```python
from build123d import *

# Parameters (mm, degrees)
F0_W     = 4.5
F0_H     = 30
F0_W_2   = 4
F1_DEPTH = 5
F2_DEPTH = 10
F3_R     = 3
F4_R     = 1
F6_DEPTH = 30


with BuildPart() as f1:
    # F0 (on Top) → F1 (new body)
    with BuildSketch(Plane.XY):
        with Locations((-4.7856509686, -8.5439818352)):
            Rectangle(F0_W, F0_H)
        with Locations((-9.0356509686, -8.5439818352)):
            Rectangle(F0_W_2, F0_H)
        with Locations((-0.5356509686, -8.5439818352)):
            Rectangle(F0_W_2, F0_H)
    extrude(amount=-F1_DEPTH)

    # F0 (on Top) → F2 (join)
    with BuildSketch(Plane.XY):
        with Locations((-9.0356509686, -8.5439818352)):
            Rectangle(F0_W_2, F0_H)
        with Locations((-0.5356509686, -8.5439818352)):
            Rectangle(F0_W_2, F0_H)
    extrude(amount=F2_DEPTH)

    # F3
    f3_edges = [f1.edges().sort_by_distance(p)[0] for p in [
        (1.464349, -8.543982, -5),
        (-11.035651, -8.543982, -5),
    ]]
    fillet(f3_edges, radius=F3_R)

    # F4
    f4_edges = [f1.edges().sort_by_distance(p)[0] for p in [
        (-7.035651, -8.543982, 10),
        (-11.035651, -8.543982, 10),
        (1.464349, -8.543982, 10),
        (-2.535651, -8.543982, 10),
    ]]
    fillet(f4_edges, radius=F4_R)

    # F5 (on face) → F6 (join)
    with BuildSketch(Plane.XZ.offset(23.5439818352)):
        with BuildLine():
            Line((-2.5356509686, 6.1144679785), (-2.5356509686, 8.4431599826))
            add(Edge.make_bspline(
                [(-2.5356509686, 8.4431599826), (-2.7152575285, 8.0569054131), (-2.9551929536, 7.2933215725), (-2.7169880221, 6.5044440771), (-2.5356509686, 6.1144679785)],
                knots=[0, 0, 0, 0, 0.49760282, 1, 1, 1, 1], degree=3))
        make_face()
        with BuildLine():
            Line((-7.0356509686, 8.4431599826), (-7.0356509686, 6.1144679785))
            add(Edge.make_bspline(
                [(-7.0356509686, 8.4431599826), (-6.8227021242, 8.0569054131), (-6.6496118928, 7.2933215725), (-6.8206503806, 6.5044440771), (-7.0356509686, 6.1144679785)],
                knots=[0, 0, 0, 0, 0.49760282, 1, 1, 1, 1], degree=3))
        make_face()
    extrude(amount=-F6_DEPTH)


solid = f1.part
```
Can you work these out from the model? Positions are in its coordinate system, mm. A direction names the side the tool comes from. Coordinates: 2 decimals unless noted, no trailing zeros. Loops run counter-clockwise (first coordinate to the right, second up) from the corner with the lowest first, then second, coordinate; pieces in that order, holes last.
1) Imagine slicing it at B-B on x = 0. List the corners of the cut face in (y, z) for me.
2) I need wall thicknesses on probe 1 along X at (y, z) = (-11.5, 4.5); probe 2 along Z at (x, y) = (-7, -7.5); probe 3 along X at (y, z) = (-9, 9.5). Which ranges of each line are inside material? Lowest first, please.
3) For pin 1 (2 mm diameter, centred on x = -4, y = -6.5, fed in from +Z), with a flat end and sliding along its axis, tell me the tip position at first contact or that it passes through.
4) Imagine slicing it at A-A on z = 1.25. List the corners of the cut face in (x, y) for me.
5) Thinking about a two-plate mould opening in Z: for faces 1 (the flat face through (-5, -8, -5)), 2 (the cylindrical face through (-2.25, -8.33, 9.7)), 3 (the flat face through (-7.036, -9, 3)), which applies, pulls with the +Z half, pulls with the -Z half, needs draft (parallel to the pull), parting line crosses it, or undercut?
6) Which directions (+Z, -Z, +X, -X, +Y, -Y) give clear straight access to the entire face, cutting with the end or side of a thin tool? Please do faces 4 (the flat face through (-2.536, -9, 3)), 5 (the flat face through (-11.036, -9, 3)), 6 (the cylindrical face through (-7.336, -8.334, 9.715)).
Completed:
1. outline: (-23.54, -4.58) - (6.46, -4.58) - (6.46, 10) - (-23.54, 10) - close
2. probe 1: x = -11.04 to -7.04, -2.54 to 1.46
2. probe 2: z = -5 to 0, 6.18 to 8.38
2. probe 3: x = -10.9 to -7.17, -2.4 to 1.33
3. pin 1: stops at z = 0
4. outline: (-11.04, -23.54) - (-7.04, -23.54) - (-7.04, 6.46) - (-11.04, 6.46) - close; (-2.54, -23.54) - (1.46, -23.54) - (1.46, 6.46) - (-2.54, 6.46) - close
5. face 1: pulls with the -Z half
5. face 2: pulls with the +Z half
5. face 3: undercut
6. face 4: +Y, -Y
6. face 5: +Z, -Z, -X, +Y, -Y
6. face 6: +Z, +Y, -Y
